Read the model definition and answer for the solid it produces. Units are mm, in the model's axes. Face numbers are marked on the shaded views. A direction names the side the tool comes from. Coordinates: 2 decimals unless noted, no trailing zeros. Loops run counter-clockwise (first coordinate to the right, second up) from the corner with the lowest first, then second, coordinate; pieces in that order, holes last.
Q1. The mould has two halves that part along Y. Classify the marked faces 3, 4 and 5: pulls with the +Y half, pulls with the -Y half, needs draft (parallel to the pull), parting line crosses it, or undercut.
Q2. Section C-C (x = 3) is taken. Give the vertices of the cut face in (y, z), then the cut area to 3 significant figures.
Q3. Straight lines are drawn through the part: line 1 (Y direction, x = 27, z = 0); line 2 (Z direction, x = 33.5, y = -1); line 3 (X direction, y = -12, z = 33). For each, find the intervals that lie inside material, in ascending order.
Q4. Flat-ended cylindrical pins translate along their axes: P1, Ø1.5, axis at x = 21.5, y = -2.5, coming from the -Z side; P2, Ø1.5, axis at x = 6, y = 6, coming from the -Z side; P3, Ø3, axis at x = 26, y = 23.5, coming from the -Z side. Find the tip coordinate at first contact, or state that the pin passes through.
Q5. Section A-A (y = 0) is taken. Give the vertices of the cut face in (x, z).
Q6. Which of the six approach directions +Z, -Z, +X, -X, +Y, -Y give full straight-line access (tool end or side, diameter ignored) to the marked faces 1 and 2?
Q7. Section B-B (z = 0) is taken. Give the vertices of the cut face in (x, y).
Q8. Section D-D (x = 32) is taken. Give the vertices of the cut face in (y, z).
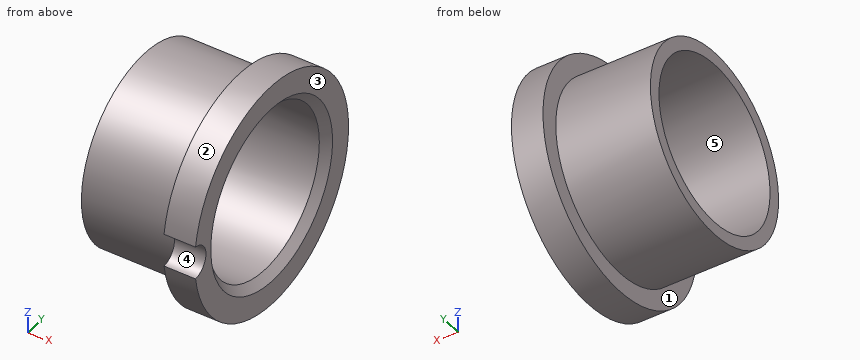
from build123d import *

# Parameters (mm, degrees)
SKETCH2_R             = 30
BOSS_EXTRUDE1_DEPTH   = 30
SKETCH3_R             = 36
BOSS_EXTRUDE2_DEPTH   = 10
SKETCH4_R             = 26
CUT_EXTRUDE1_DEPTH    = 65.745656225
CHAMFER1_SIZE         = 2.5
D_GAGEMENT_M101_D     = 10.5
D_GAGEMENT_M101_DEPTH = 20
D_GAGEMENT_M101_TIP   = 3.15451825


with BuildPart() as part:
    # Sketch2 → Boss-Extrude1 (new body)
    with BuildSketch(Plane(origin=(0, 0, 0), x_dir=(0, 0, -1), z_dir=(1, 0, 0))):
        Circle(SKETCH2_R)
    extrude(amount=BOSS_EXTRUDE1_DEPTH)

    # Sketch3 → Boss-Extrude2 (add)
    with BuildSketch(Plane(origin=(30, 0, 0), x_dir=(0, 0, -1), z_dir=(1, 0, 0))):
        Circle(SKETCH3_R)
    extrude(amount=BOSS_EXTRUDE2_DEPTH)

    # Sketch4 → Cut-Extrude1 (cut, through all)
    with BuildSketch(Plane(origin=(40, 0, 0), x_dir=(0, 0, -1), z_dir=(1, 0, 0))):
        Circle(SKETCH4_R)
    extrude(amount=-CUT_EXTRUDE1_DEPTH, mode=Mode.SUBTRACT)

    # Chamfer1
    chamfer1_edges = [part.edges().sort_by_distance(p)[0] for p in [
        (40, 0, 26),
    ]]
    chamfer(chamfer1_edges, length=CHAMFER1_SIZE)

    # Dégagement M101
    with Locations(Plane(origin=(40, 0, 0), x_dir=(0, 0, -1), z_dir=(1, 0, 0))):
        with Locations((0, -36)):
            Hole(D_GAGEMENT_M101_D / 2, depth=D_GAGEMENT_M101_DEPTH)
            with Locations((0, 0, -(D_GAGEMENT_M101_DEPTH + D_GAGEMENT_M101_TIP / 2))):  # 118° drill point
                Cone(0, D_GAGEMENT_M101_D / 2, D_GAGEMENT_M101_TIP, mode=Mode.SUBTRACT)


solid = part.part
Numbers:
1. face 3: needs draft
1. face 4: pulls with the -Y half
1. face 5: undercut
2. outline: circle Ø60 at (0, 0); hole circle Ø52 at (0, 0)
2. area: 704 mm2
3. line 1: y = -30 to -26, 26 to 30
3. line 2: z = -35.99 to -25.98, 25.98 to 35.99
3. line 3: x = 30 to 40
4. P1: stops at z = -29.95
4. P2: stops at z = -29.54
4. P3: stops at z = -20.4
5. outline: (0, -30) - (30, -30) - (30, -36) - (40, -36) - (40, -28.5) - (37.5, -26) - (0, -26) - close; (0, 26) - (37.5, 26) - (40, 28.5) - (40, 36) - (30, 36) - (30, 30) - (0, 30) - close
6. face 1: -X
6. face 2: +X, -X
7. outline: (0, -30) - (30, -30) - (30, -30.75) - (40, -30.75) - (40, -28.5) - (37.5, -26) - (0, -26) - close; (0, 26) - (37.5, 26) - (40, 28.5) - (40, 36) - (30, 36) - (30, 30) - (0, 30) - close
8. outline: (-35.62, -5.24) arc R36 ccw (long way) to (-35.62, 5.24) arc R5.25 cw to start; hole circle Ø52 at (0, 0)
